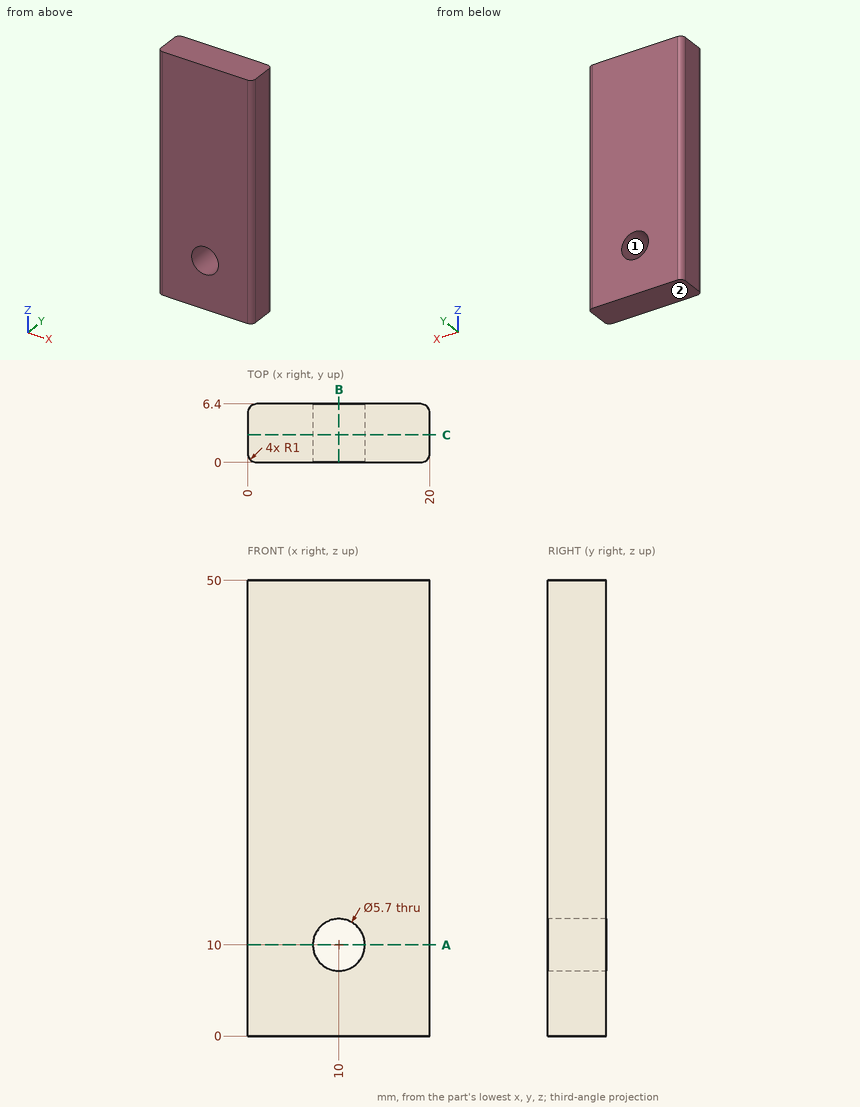
Verification items for this drawing (mm, ordinates from the low corner). Round coordinates to 2 decimals unless told otherwise and drop trailing zeros. Order: outer loops, then holes, each group sorted by start corner. A loop starts at its lowest first (then second) coordinate and runs counter-clockwise, first axis right, second up. Notation, with made-up numbers: M 10.25,16.25 L 43.25,16.25 A6 ccw 43.25,25.25 Z; hole C -24.75,39.25 d8. An arc over 180 degrees is marked long. Answer in a Markdown table with one row per item. Add a question column.
Item 1: Sectioned sample at B-B, the plane x = 10. Enter the section's corners in (y, z).
Item 2: Sectioned sample at C-C, the plane y = 3. Enter the section's corners in (x, z), plus the area to 3 significant figures.
Item 3: Draft check along X on the marked faces 1 and 2. Enter one of: released by +X, released by -X, zero draft, split by the parting line, or undercut.
Item 4: Material ranges on L1, parallel to X at y = 4.5, z = 10; L2, parallel to X at y = 0.5, z = 10.5; L3, parallel to Z at x = 12.25, y = 5, recorded low to high. Write a range as [from, to].
Item 5: Depth check by flat-ended pin: pin 1 Ø3 at (x, y) = (8, 3.5) entering from -Z. Enter the tip coordinate at first touch or a pass-through.
Item 6: Sectioned sample at A-A, the plane z = 10. Enter the section's corners in (x, y), plus the area to 3 significant figures.
Filled in:
| question | item | result |
|---|---|---|
| 1 | outline | M 0,0 L 6.4,0 L 6.4,7.15 L 0,7.15 Z; M 0,12.85 L 6.4,12.85 L 6.4,50 L 0,50 Z |
| 2 | outline | M 0,0 L 20,0 L 20,50 L 0,50 Z; hole C 10,10 d5.7 |
| 2 | area | 974 mm² |
| 3 | face 1 | undercut |
| 3 | face 2 | zero draft |
| 4 | L1 | x = [0, 7.15], [12.85, 20] |
| 4 | L2 | x = [0.13, 7.19], [12.81, 19.87] |
| 4 | L3 | z = [0, 8.25], [11.75, 50] |
| 5 | pin 1 | stops at z = 0 |
| 6 | outline | M 0,1 A1 ccw 1,0 L 7.15,0 L 7.15,6.4 L 1,6.4 A1 ccw 0,5.4 Z; M 12.85,0 L 19,0 A1 ccw 20,1 L 20,5.4 A1 ccw 19,6.4 L 12.85,6.4 Z |
| 6 | area | 90.7 mm² |
